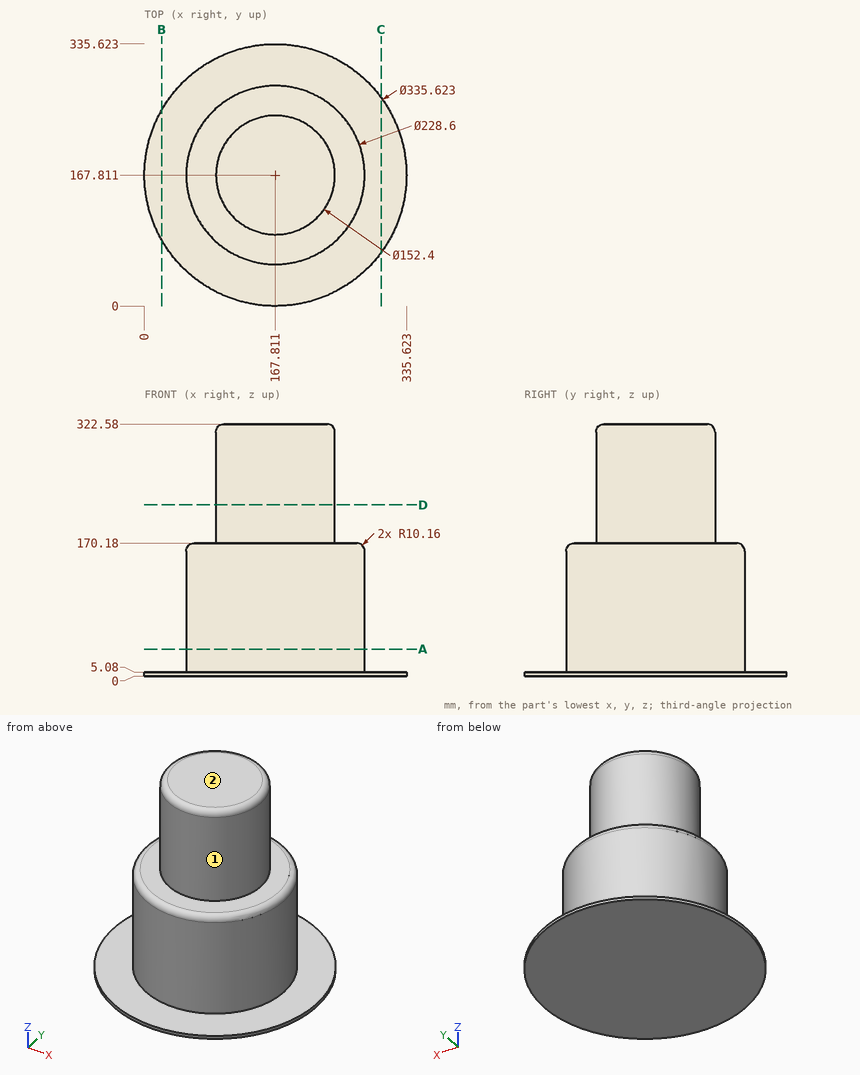
Check sheet for the drawn part. Datum: minimum x, y, z corner. Units: mm. A direction names the side the tool comes from. Round coordinates to 2 decimals unless told otherwise and drop trailing zeros. Write each loop counter-clockwise with the first axis right and the second up, starting at its lowest first coordinate (ties: lowest second). Pieces come first, ordered by that corner, then holes. Notation, with made-up numbers: (7, 83.25) - (12, 83.25) arc R14 cw to (12, 107.25) - close; hole circle Ø11 at (42.5, -26). An arc over 180 degrees is marked (long way). Return JSON: item names as keys, results as strings.
Q1. Access from +Z, -Z, +X, -X, +Y, -Y to the whole of each face (thin tool, end or side, straight path). Record for the marked faces 1 and 2.
Returned:
{"face 1": "+Z", "face 2": "+Z, +X, -X, +Y, -Y"}
Q2. Cross-section at B-B (x = 22). Record the boundary of the cut face in (y, z), then the cut area to 3 significant figures.
Returned:
{"outline": "(84.75, 0) - (250.88, 0) - (250.88, 5.08) - (84.75, 5.08) - close", "area": "844 mm²"}
Q3. Scan lines: L1, parallel to Z at x = 241, y = 290; L2, parallel to Z at x = 173.5, y = 261; L3, parallel to X at y = 131, z = 70.5. Record each from-to range of solid material in increasing order. Write a range as from..to.
Returned:
{"L1": "z = 0..5.08", "L2": "z = 0..170.18", "L3": "x = 59.6..276.02"}
Q4. Depth check by flat-ended pin: P1, Ø5, axis at y = 259, z = 55.5, coming from the -X side; P2, Ø6, axis at y = 161.5, z = 243.5, coming from the +X side; P3, Ø4, axis at x = 119.5, z = 125, coming from the -Y side. Enter the tip coordinate at first touch or a pass-through.
Returned:
{"P1": "stops at x = 95.71", "P2": "stops at x = 243.94", "P3": "stops at y = 63.31"}
Q5. Cross-section at D-D (z = 219). Record the boundary of the cut face in (x, y).
Returned:
{"outline": "circle Ø152.4 at (167.81, 167.81)"}
Q6. Cross-section at C-C (x = 303). Record the boundary of the cut face in (y, z), then the cut area to 3 significant figures.
Returned:
{"outline": "(68.39, 0) - (267.23, 0) - (267.23, 5.08) - (68.39, 5.08) - close", "area": "1,010 mm²"}
Q7. Cross-section at A-A (z = 34.5). Record the boundary of the cut face in (x, y), then the cut area to 3 significant figures.
Returned:
{"outline": "circle Ø228.6 at (167.81, 167.81)", "area": "41,000 mm²"}
